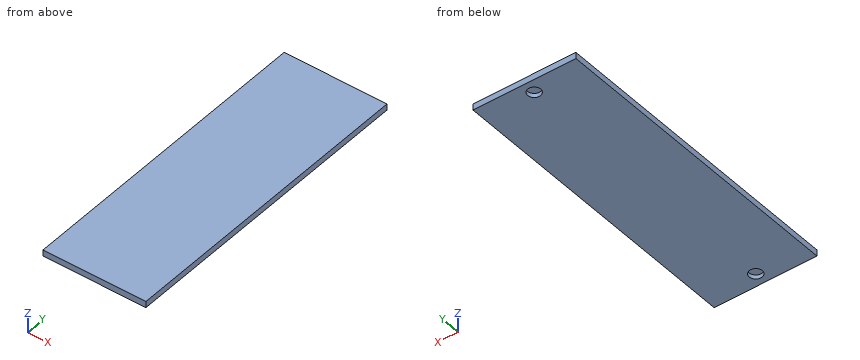
```python
from build123d import *

# Parameters (mm, degrees)
SKETCH_W     = 49.4
SKETCH_H     = 148
PAD_DEPTH    = 3
SKETCH001_R  = 3.1
POCKET_DEPTH = 2


with BuildPart() as part:
    # Sketch → Pad (new body)
    with BuildSketch(Plane.XY):
        with Locations((24.7, 74)):
            Rectangle(SKETCH_W, SKETCH_H)
    extrude(amount=PAD_DEPTH)

    # Sketch001 → Pocket (cut)
    with BuildSketch(Plane.XY):
        with Locations((24.7, 6)):
            Circle(SKETCH001_R)
        with Locations((24.7, 142)):
            Circle(SKETCH001_R)
    extrude(amount=POCKET_DEPTH, mode=Mode.SUBTRACT)


solid = part.part
```
Geometry check sheet. Reference: the model listing, model coordinates, mm. Coordinates: 2 decimals unless noted, no trailing zeros. Loops run counter-clockwise (first coordinate to the right, second up) from the corner with the lowest first, then second, coordinate; pieces in that order, holes last. Notation, with made-up numbers: (41, 24) - (59, 24) arc R30 ccw to (59, 61) - close; hole circle Ø1 at (65, -29). An arc over 180 degrees is marked (long way). One line per item, written item: value. Start each with the question number.
(1) Cross-section at A-A on x = 24.7. Enter the section's corners in (y, z).
(2) Depth check by flat-ended pin: P1, Ø12, axis at x = 39.5, y = 107, coming from the -Z side; P2, Ø1.9, axis at x = 25, y = 143.5, coming from the -Z side. Enter the tip coordinate at first touch or a pass-through.
(3) Material ranges on line 1 (Y direction, x = 24.7, z = 0.65); line 2 (X direction, y = 142, z = 1.15); line 3 (Y direction, x = 26, z = 1.9), recorded low to high. Write a range as [from, to].
(4) Cross-section at B-B on y = 142. Enter the section's corners in (x, z).
Results below:
1. outline: (0, 0) - (2.9, 0) - (2.9, 2) - (9.1, 2) - (9.1, 0) - (138.9, 0) - (138.9, 2) - (145.1, 2) - (145.1, 0) - (148, 0) - (148, 3) - (0, 3) - close
2. P1: stops at z = 0
2. P2: stops at z = 2
3. line 1: y = [0, 2.9], [9.1, 138.9], [145.1, 148]
3. line 2: x = [0, 21.6], [27.8, 49.4]
3. line 3: y = [0, 3.19], [8.81, 139.19], [144.81, 148]
4. outline: (0, 0) - (21.6, 0) - (21.6, 2) - (27.8, 2) - (27.8, 0) - (49.4, 0) - (49.4, 3) - (0, 3) - close
